Job drawing, mm, ordinate dimensions from the low corner. One solid piece. A direction names the side the tool comes from. Round coordinates to 2 decimals unless told otherwise and drop trailing zeros. Write each loop counter-clockwise with the first axis right and the second up, starting at its lowest first coordinate (ties: lowest second). Pieces come first, ordered by that corner, then holes. Notation, with made-up numbers: M -12.75,54.5 L 24.25,54.5 A20 ccw 24.25,80.5 Z; hole C 21,22.25 d9. An arc over 180 degrees is marked long. Write each question's results on one line, items separated by ' | '. Start each with the question number.
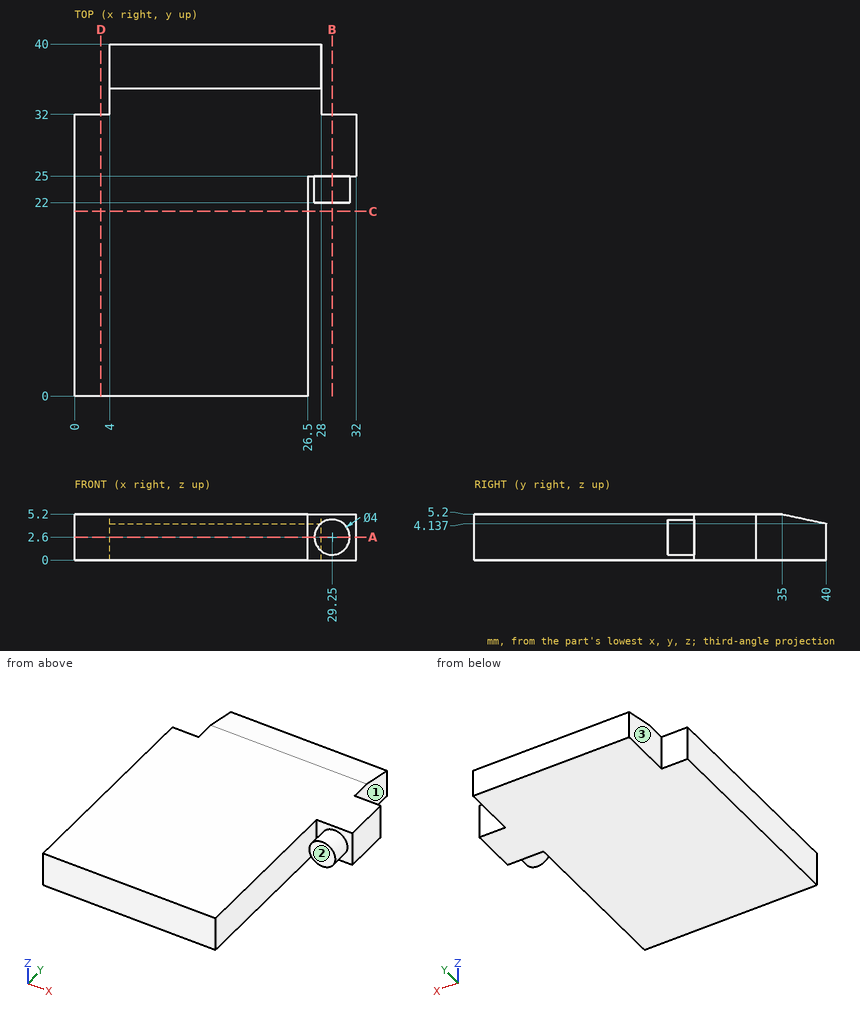
1) Saw through at A-A, the plane z = 2.6. Write the cut outline in (x, y).
2) Drop flat-ended pins along their axis: pin 1 Ø3 at (x, z) = (29.5, 2.5) entering from -Y; pin 2 Ø1.2 at (x, z) = (3, 2.5) entering from +Y; pin 3 Ø2.5 at (y, z) = (17, 4) entering from +X. Give the stop position or say it passes through.
3) Saw through at C-C, the plane y = 21. Write the cut outline in (x, z).
4) Wall check: line 1 along X through (y, z) = (14, 3.8); line 2 along Y through (x, z) = (27.5, 1.95); line 3 along Y through (x, z) = (31, 2.05). Give the ranges that are in metal, low to high. Write a range as from..to.
5) Saw through at B-B, the plane x = 29.25. Write the cut outline in (y, z), plus the area to 3 significant figures.
6) Saw through at D-D, the plane x = 3. Write the cut outline in (y, z).
7) 3-axis set-ups, long thin cutter, end or side, ignore diameter. For the marked faces 1, 2 and 3: which of +Z, -Z, +X, -X, +Y, -Y reach the whole face in a straight line?
Filled sheet:
1) outline: M 0,0 L 26.5,0 L 26.5,25 L 27.25,25 L 27.25,22 L 31.25,22 L 31.25,25 L 32,25 L 32,32 L 28,32 L 28,40 L 4,40 L 4,32 L 0,32 Z
2) pin 1: stops at y = 22 | pin 2: stops at y = 32 | pin 3: stops at x = 26.5
3) outline: M 0,0 L 26.5,0 L 26.5,5.2 L 0,5.2 Z
4) line 1: x = 0..26.5 | line 2: y = 22..40 | line 3: y = 22..32
5) outline: M 22,0.6 L 25,0.6 L 25,0 L 32,0 L 32,5.2 L 25,5.2 L 25,4.6 L 22,4.6 Z | area: 48.4 mm^2
6) outline: M 0,0 L 32,0 L 32,5.2 L 0,5.2 Z
7) face 1: +Z, -Z, +X, +Y | face 2: +Z, -Z, +X, -Y | face 3: +Z, -Z, -X, +Y
